The model under review builds one solid part; all positions refer to its coordinate system, in mm. Give positions to 0.01 mm unless a question says otherwise; leave off trailing zeros. Loops run counter-clockwise (first coordinate to the right, second up) from the corner with the lowest first, then second, coordinate; pieces in that order, holes last. Notation, with made-up numbers: M 12.25,3 L 20.25,3 A36 cw 20.25,42 Z; hole C 56.25,30 d1. An arc over 180 degrees is marked long. Return JSON: item names as keys, results as strings.
```python
from build123d import *

# Parameters (mm, degrees)
F0_R     = 3
F0_R_2   = 2
F1_DEPTH = 10
F0_R_3   = 5
F2_DEPTH = 2
F3_R     = 0.5


with BuildPart() as f1:
    # F0 (on Top) → F1 (new body)
    with BuildSketch(Plane.XY):
        Circle(F0_R)
        Circle(F0_R_2, mode=Mode.SUBTRACT)
    extrude(amount=F1_DEPTH)

    # F0 (on Top) → F2 (join)
    with BuildSketch(Plane.XY):
        Circle(F0_R_3)
        Circle(F0_R, mode=Mode.SUBTRACT)
    extrude(amount=F2_DEPTH)

    # F3
    f3_edges = [f1.edges().sort_by_distance(p)[0] for p in [
        (-5, 0, 0),
        (-2, 0, 0),
    ]]
    fillet(f3_edges, radius=F3_R)


solid = f1.part
```
1) Consider section C-C on z = 1.75. Write out the cut boundary in (x, y), then the cut area to 3 significant figures.
From the geometry:
{"outline": "C 0,0 d10; hole C 0,0 d4", "area": "66.0 mm²"}
2) Insertion check: pin 1 (6 mm diameter, centred on x = -4, z = 3, fed in from -Y); pin 2 (2 mm diameter, centred on x = -2, z = 5.5, fed in from +Y); pin 3 (4.5 mm diameter, centred on x = 0, y = 0, fed in from -Z). Each pin has a flat end and moves straight along its axis. Give the tip position at first contact, or say it passes through.
From the geometry:
{"pin 1": "y = -4.86", "pin 2": "y = 2.83", "pin 3": "z = 0.07"}
3) Consider section A-A on y = 0. Write out the cut boundary in (x, z), then the cut area to 3 significant figures.
From the geometry:
{"outline": "M -5,0.5 A0.5 ccw -4.5,0 L -2.5,0 A0.5 ccw -2,0.5 L -2,10 L -3,10 L -3,2 L -5,2 Z; M 2,0.5 A0.5 ccw 2.5,0 L 4.5,0 A0.5 ccw 5,0.5 L 5,2 L 3,2 L 3,10 L 2,10 Z", "area": "27.8 mm²"}
4) The part is to be moulded in two halves that separate along Y. For faces 1 (the face through (0, -2, 5)), 2 (the face through (-0.1, -3.3, 2)), 3 (the face through (-3, 0, 6)), say which applies: released by +Y, released by -Y, zero draft, split by the parting line, or undercut.
From the geometry:
{"face 1": "undercut", "face 2": "zero draft", "face 3": "split by the parting line"}
5) Wall thickness on L1, parallel to Y at x = 0, z = 3.5; L2, parallel to Z at x = -3.25, y = -2.5; L3, parallel to X at y = -0.25, z = 8: over which ranges is each line inside the solid? List them lowest first. Write a range as from..to.
From the geometry:
{"L1": "-3..-2, 2..3", "L2": "0..2", "L3": "-2.99..-1.98, 1.98..2.99"}
6) Consider section D-D on z = 3.5. Write out the cut boundary in (x, y).
From the geometry:
{"outline": "C 0,0 d6; hole C 0,0 d4"}
